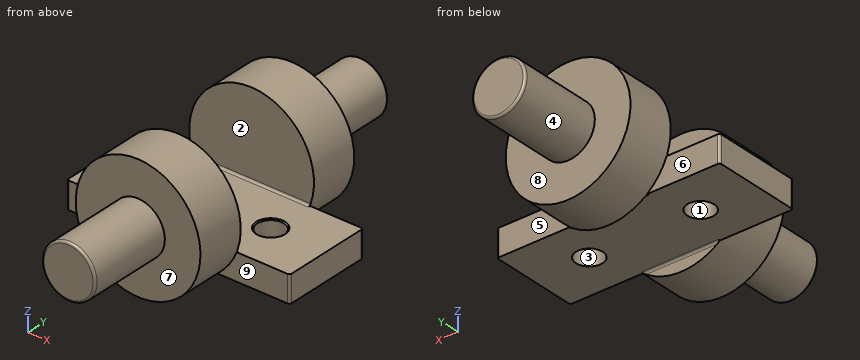
from build123d import *

# Parameters (mm, degrees)
CROQUIS1_R                 = 6
SALIENTE_EXTRUIR1_DEPTH    = 19
CROQUIS2_R                 = 14
SALIENTE_EXTRUIR2_DEPTH    = 11
CROQUIS5_W                 = 50
CROQUIS5_H                 = 6
SALIENTE_EXTRUIR6_DEPTH    = 20
CROQUIS6_R                 = 14
SALIENTE_EXTRUIR7_DEPTH    = 11
SALIENTE_EXTRUIR8_START    = 19
CROQUIS7_R                 = 6
SALIENTE_EXTRUIR8_DEPTH    = 19
CORTAR_EXTRUIR2_DEPTH      = 69.607579756
CORTAR_EXTRUIR2_DEPTH_BACK = 69.607579756
CROQUIS9_R                 = 3
REDONDEO2_R                = 0.5
CHAFL_N1_SIZE              = 0.25


with BuildPart() as part:
    # Croquis1 → Saliente-Extruir1 (new body)
    with BuildSketch(Plane(origin=(0, 0, 0), x_dir=(1, 0, 0), z_dir=(0, 1, 0))):
        with Locations(Location((0, 0, 0), (0, 0, 270))):
            Circle(CROQUIS1_R)
    extrude(amount=-SALIENTE_EXTRUIR1_DEPTH)

    # Croquis2 → Saliente-Extruir2 (add)
    with BuildSketch(Plane(origin=(0, 0, 0), x_dir=(1, 0, 0), z_dir=(0, 1, 0))):
        with Locations(Location((0, 0, 0), (0, 0, 270))):
            Circle(CROQUIS2_R)
    extrude(amount=SALIENTE_EXTRUIR2_DEPTH)

    # Croquis5 → Saliente-Extruir6 (add)
    with BuildSketch(Plane(origin=(0, 11, 0), x_dir=(1, 0, 0), z_dir=(0, 1, 0))):
        with Locations((0, 8)):
            Rectangle(CROQUIS5_W, CROQUIS5_H)
    extrude(amount=SALIENTE_EXTRUIR6_DEPTH)

    # Croquis6 → Saliente-Extruir7 (add)
    with BuildSketch(Plane(origin=(0, 31, 0), x_dir=(1, 0, 0), z_dir=(0, 1, 0))):
        with Locations(Location((0, 0, 0), (0, 0, 128.213210702))):
            Circle(CROQUIS6_R)
    extrude(amount=SALIENTE_EXTRUIR7_DEPTH)

    # Croquis7 → Saliente-Extruir8 (add)
    with BuildSketch(Plane(origin=(0, 42, 0), x_dir=(1, 0, 0), z_dir=(0, 1, 0)).offset(SALIENTE_EXTRUIR8_START)):
        with Locations(Location((0, 0, 0), (0, 0, 270))):
            Circle(CROQUIS7_R)
    extrude(amount=-SALIENTE_EXTRUIR8_DEPTH)

    # Croquis9 → Cortar-Extruir2 (cut, two sides: drawn at the far end of the back side and taken through both)
    with BuildSketch(Plane.XY.offset(-5).offset(-CORTAR_EXTRUIR2_DEPTH_BACK)):
        with Locations((-12.5, 21)):
            Circle(CROQUIS9_R)
        with Locations((12.5, 21)):
            Circle(CROQUIS9_R)
    extrude(amount=CORTAR_EXTRUIR2_DEPTH + CORTAR_EXTRUIR2_DEPTH_BACK, mode=Mode.SUBTRACT)

    # Redondeo2
    # the kernel refuses this fillet: 0.5 mm, written as the material it adds along each edge
    with BuildSketch(Plane(origin=(9.910254038, 11, -11), x_dir=(0, 0, -1), z_dir=(-1, 0, 0))) as redondeo2_piece_1_section:
        with BuildLine():
            CenterArc((REDONDEO2_R, -REDONDEO2_R), REDONDEO2_R, 90, 90)
            Line((0, -REDONDEO2_R), (0, 0))
            Line((0, 0), (REDONDEO2_R, 0))
        make_face()
    redondeo2_piece_1 = extrude(amount=19.820508076, mode=Mode.PRIVATE)
    redondeo2_piece_1 = redondeo2_piece_1 & Plane(origin=(0, 11.11248229, 0), x_dir=(0, 0, 1), z_dir=(0, -1, 0)) * Cylinder(14, 42, mode=Mode.PRIVATE)
    add(redondeo2_piece_1)
    with BuildSketch(Plane(origin=(-14.326696831, 11, -5), x_dir=(0, 0, 1), z_dir=(1, 0, 0))) as redondeo2_piece_2_section:
        with BuildLine():
            CenterArc((REDONDEO2_R, -REDONDEO2_R), REDONDEO2_R, 90, 90)
            Line((0, -REDONDEO2_R), (0, 0))
            Line((0, 0), (REDONDEO2_R, 0))
        make_face()
    redondeo2_piece_2 = extrude(amount=28.653393661, mode=Mode.PRIVATE)
    redondeo2_piece_2 = redondeo2_piece_2 & Plane(origin=(0, 11.111538065, 0), x_dir=(0, 0, 1), z_dir=(0, -1, 0)) * Cylinder(14, 60, mode=Mode.PRIVATE)
    add(redondeo2_piece_2)
    with BuildSketch(Plane(origin=(-14.326696831, 31, -5), x_dir=(0, -1, 0), z_dir=(1, 0, 0))) as redondeo2_piece_3_section:
        with BuildLine():
            CenterArc((REDONDEO2_R, -REDONDEO2_R), REDONDEO2_R, 90, 90)
            Line((0, -REDONDEO2_R), (0, 0))
            Line((0, 0), (REDONDEO2_R, 0))
        make_face()
    redondeo2_piece_3 = extrude(amount=28.653393661, mode=Mode.PRIVATE)
    redondeo2_piece_3 = redondeo2_piece_3 & Plane(origin=(0, 30.888461941, 0), x_dir=(-0.6185895741353322, 0, -0.7857142857114591), z_dir=(0, -1, 0)) * Cylinder(14, 60, mode=Mode.PRIVATE)
    add(redondeo2_piece_3)
    with BuildSketch(Plane(origin=(9.910254038, 31, -11), x_dir=(0, -1, 0), z_dir=(-1, 0, 0))) as redondeo2_piece_4_section:
        with BuildLine():
            CenterArc((REDONDEO2_R, -REDONDEO2_R), REDONDEO2_R, 90, 90)
            Line((0, -REDONDEO2_R), (0, 0))
            Line((0, 0), (REDONDEO2_R, 0))
        make_face()
    redondeo2_piece_4 = extrude(amount=19.820508076, mode=Mode.PRIVATE)
    redondeo2_piece_4 = redondeo2_piece_4 & Plane(origin=(0, 30.887517705, 0), x_dir=(-0.6185895741353322, 0, -0.7857142857114591), z_dir=(0, -1, 0)) * Cylinder(14, 42, mode=Mode.PRIVATE)
    add(redondeo2_piece_4)
    # the kernel refuses this fillet: 0.5 mm, written as the material it takes off along each edge
    with BuildSketch(Plane(origin=(0, -19, 0), x_dir=(0, 0, 1), z_dir=(-1, 0, 0))) as redondeo2_2_piece_1:
        with BuildLine():
            CenterArc((6 - REDONDEO2_R, REDONDEO2_R), REDONDEO2_R, 270, 90)
            Line((6 - REDONDEO2_R, 0), (6, 0))
            Line((6, 0), (6, REDONDEO2_R))
        make_face()
    revolve(axis=Axis((0, -19, 0), (0, 1, 0)), mode=Mode.SUBTRACT)
    with BuildSketch(Plane(origin=(0, 61, 0), x_dir=(0, 0, 1), z_dir=(-1, 0, 0))) as redondeo2_2_piece_2:
        with BuildLine():
            CenterArc((6 - REDONDEO2_R, -REDONDEO2_R), REDONDEO2_R, 0, 90)
            Line((6 - REDONDEO2_R, 0), (6, 0))
            Line((6, 0), (6, -REDONDEO2_R))
        make_face()
    revolve(axis=Axis((0, 61, 0), (0, 1, 0)), mode=Mode.SUBTRACT)
    with BuildSketch(Plane(origin=(25, 11, -3.75), x_dir=(-1, 0, 0), z_dir=(0, 0, -1)), Plane(origin=(25, 31, -3.75), x_dir=(0, -1, 0), z_dir=(0, 0, -1)), Plane(origin=(-25, 11, -12.25), x_dir=(1, 0, 0), z_dir=(0, 0, 1)), Plane(origin=(-25, 31, -12.25), x_dir=(0, -1, 0), z_dir=(0, 0, 1))) as redondeo2_2_piece_3:
        with BuildLine():
            CenterArc((REDONDEO2_R, REDONDEO2_R), REDONDEO2_R, 180, 90)
            Line((0, REDONDEO2_R), (0, 0))
            Line((0, 0), (REDONDEO2_R, 0))
        make_face()
    extrude(amount=8.5, mode=Mode.SUBTRACT)

    # Chaflán1
    chafl_n1_edges = [part.edges().sort_by_distance(p)[0] for p in [
        (-15.5, 21, -5),
        (9.5, 21, -5),
    ]]
    chamfer(chafl_n1_edges, length=CHAFL_N1_SIZE)


solid = part.part
Check sheet for the modelled part. Datum: model origin and axes. Units: mm. Face numbers are marked on the shaded views. A direction names the side the tool comes from. Give positions to 0.01 mm unless a question says otherwise; leave off trailing zeros. Loops run counter-clockwise (first coordinate to the right, second up) from the corner with the lowest first, then second, coordinate; pieces in that order, holes last. Notation, with made-up numbers: M -31,82 L 5,82 A28 ccw 5,120 Z; hole C 40.5,41 d8. An arc over 180 degrees is marked long. Return JSON: item names as keys, results as strings. Group by question number.
1. Mould release check, pull along X, two halves, no side actions. Record for the marked faces 1, 2, 3 and 4: released by +X, released by -X, zero draft, split by the parting line, or undercut.
2. Cross-section at C-C on z = -7.75. Record the boundary of the cut face in (x, y).
3. Cross-section at D-D on y = 7. Record the boundary of the cut face in (x, z), plus the area to 3 significant figures.
4. Thickness scan on L1, parallel to X at y = 21, z = -7.45; L2, parallel to Y at x = 12.5, z = -9; L3, parallel to Y at x = 12, z = 4.5. Record the ranges inside material, lowest first.
5. Go/stop test with flat-tipped pins: pin 1 (12 mm diameter, centred on x = 6.5, y = 14, fed in from +Z); pin 2 (5.5 mm diameter, centred on x = 6.5, z = 8.5, fed in from +Y); pin 3 (1.8 mm diameter, centred on x = -14.5, z = -8.5, fed in from -Y). Record where each tip stops, or that it passes through.
6. Cross-section at A-A on z = 0. Record the boundary of the cut face in (x, y), plus the area to 3 significant figures.
7. Cross-section at B-B on x = 0. Record the boundary of the cut face in (y, z), plus the area to 3 significant figures.
8. Tool access check on the marked faces 5, 6, 7, 8 and 9. Record the directions out of +Z, -Z, +X, -X, +Y, -Y that give a thin tool (end or side, any length) a straight path to the whole face; none if there is none.
Return value:
{
 "1": {"face 1": "undercut", "face 2": "zero draft", "face 3": "undercut", "face 4": "split by the parting line"},
 "2": {"outline": "M -25,11.5 A0.5 ccw -24.5,11 L -11.66,11 L -11.66,0 L 11.66,0 L 11.66,11 L 24.5,11 A0.5 ccw 25,11.5 L 25,30.5 A0.5 ccw 24.5,31 L 11.66,31 L 11.66,42 L -11.66,42 L -11.66,31 L -24.5,31 A0.5 ccw -25,30.5 Z; hole C -12.5,21 d6; hole C 12.5,21 d6"},
 "3": {"outline": "C 0,0 d28", "area": "616 mm^2"},
 "4": {"L1": "-25 to -15.5, -9.5 to 9.5, 15.5 to 25", "L2": "11 to 18, 24 to 31", "L3": "0 to 11, 31 to 42"},
 "5": {"pin 1": "z = 13.94", "pin 2": "y = 42", "pin 3": "y = 11"},
 "6": {"outline": "M -14,0 L -6,0 L -6,-18.5 A0.5 ccw -5.5,-19 L 5.5,-19 A0.5 ccw 6,-18.5 L 6,0 L 14,0 L 14,11 L -14,11 Z; M -14,31 L 14,31 L 14,42 L 6,42 L 6,60.5 A0.5 ccw 5.5,61 L -5.5,61 A0.5 ccw -6,60.5 L -6,42 L -14,42 Z", "area": "1,070 mm^2"},
 "7": {"outline": "M -19,-5.5 A0.5 ccw -18.5,-6 L 0,-6 L 0,-14 L 11,-14 L 11,-11.5 A0.5 cw 11.5,-11 L 30.5,-11 A0.5 cw 31,-11.5 L 31,-14 L 42,-14 L 42,-6 L 60.5,-6 A0.5 ccw 61,-5.5 L 61,5.5 A0.5 ccw 60.5,6 L 42,6 L 42,14 L 31,14 L 31,-4.5 A0.5 cw 30.5,-5 L 11.5,-5 A0.5 cw 11,-4.5 L 11,14 L 0,14 L 0,6 L -18.5,6 A0.5 ccw -19,5.5 Z", "area": "1,190 mm^2"},
 "8": {"face 5": "-Z, +X, +Y", "face 6": "-Z, -X, +Y", "face 7": "-Y", "face 8": "+Y", "face 9": "-Z, +X, -Y"}
}
